```python
from build123d import *

# Parameters (mm, degrees)
F0_R     = 6.9
F0_R_2   = 2.45
F1_DEPTH = 6
F0_R_3   = 1.7
F2_DEPTH = 1.5
F3_R     = 0.5


with BuildPart() as f1:
    # F0 (on Top) → F1 (new body)
    with BuildSketch(Plane.XY):
        Circle(F0_R)
        Circle(F0_R_2, mode=Mode.SUBTRACT)
    extrude(amount=F1_DEPTH)

    # F0 (on Top) → F2 (join)
    with BuildSketch(Plane.XY):
        Circle(F0_R_2)
        Circle(F0_R_3, mode=Mode.SUBTRACT)
    extrude(amount=F2_DEPTH)

    # F3
    f3_edges = [f1.edges().sort_by_distance(p)[0] for p in [
        (-6.9, 0, 6),
        (-6.9, 0, 0),
    ]]
    fillet(f3_edges, radius=F3_R)


solid = f1.part
```
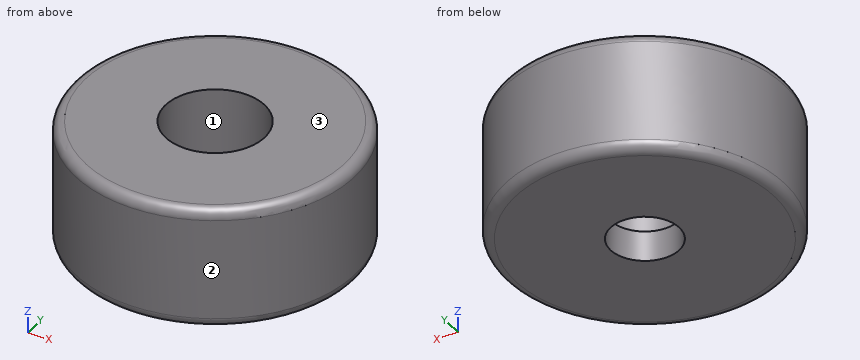
Source: CAD feature listing. Evaluate the final solid. Frame: model axes, mm. Face numbers are marked on the shaded views. Round coordinates to 2 decimals unless told otherwise and drop trailing zeros. Write each loop counter-clockwise with the first axis right and the second up, starting at its lowest first coordinate (ties: lowest second). Pieces come first, ordered by that corner, then holes. Notation, with made-up numbers: M -23.75,79.25 L 7.25,79.25 A17 ccw 7.25,97.25 Z; hole C 81.5,46.5 d2. An arc over 180 degrees is marked long. Answer as a JSON object with one key per item and string values. Group by question number.
(1) Section query A-A on y = 0. Output: boundary loops of the cut face in (x, z).
(2) Mould query, pull axis X, two halves, no side actions, for the marked faces 1, 2 and 3. Classes: +X half, -X half, draft (parallel to the pull), parting line (faces both ways), or undercut.
(3) Ray query, line 1 (Y direction, x = 0, z = 2.65); line 2 (Y direction, x = 0, z = 0.45); line 3 (X direction, y = 0.75, z = 2.75). Return the intervals inside material, ascending. Write a range as [from, to].
(4) Section query C-C on z = 4.1. Output: boundary loops of the cut face in (x, y).
(5) First-contact query: pin 1 (3 mm diameter, centred on y = -0.5, z = 3, fed in from -X); pin 2 (1 mm diameter, centred on x = -1.5, y = 0, fed in from +Z); pin 3 (3 mm diameter, centred on x = 0, y = 0, fed in from +Z). Flat tips, straight axial feed; report the tip coordinate or a pass-through.
(6) Section query D-D on z = 0.75. Output: boundary loops of the cut face in (x, y), then the cut area to 3 significant figures.
Computed values:
{
 "1": {"outline": "M -6.9,0.5 A0.5 ccw -6.4,0 L -1.7,0 L -1.7,1.5 L -2.45,1.5 L -2.45,6 L -6.4,6 A0.5 ccw -6.9,5.5 Z; M 1.7,0 L 6.4,0 A0.5 ccw 6.9,0.5 L 6.9,5.5 A0.5 ccw 6.4,6 L 2.45,6 L 2.45,1.5 L 1.7,1.5 Z"},
 "2": {"face 1": "undercut", "face 2": "parting line", "face 3": "draft"},
 "3": {"line 1": "[-6.9, -2.45], [2.45, 6.9]", "line 2": "[-6.9, -1.7], [1.7, 6.9]", "line 3": "[-6.86, -2.33], [2.33, 6.86]"},
 "4": {"outline": "C 0,0 d13.8; hole C 0,0 d4.9"},
 "5": {"pin 1": "x = -6.9", "pin 2": "z = 1.5", "pin 3": "through"},
 "6": {"outline": "C 0,0 d13.8; hole C 0,0 d3.4", "area": "140 mm^2"}
}
